Solid Edge part; units mm, degrees
sketch "Sketch1" plane through (0, 0, 0) normal (0, 0, 1) x (1, 0, 0)
  circle A0 centre (0, 0) radius 6
extrude "Protrusion1" add sketch "Sketch1" along normal mid plane 30
sketch "Sketch2" plane through (0, 0, 15) normal (0, 0, 1) x (1, 0, 0)
  line L0 (-9.9593, 5.75) -> (-9.9593, -5.75)
  line L1 (-9.9593, -5.75) -> (0, -11.5)
  line L2 (0, -11.5) -> (9.9593, -5.75)
  line L3 (9.9593, -5.75) -> (9.9593, 5.75)
  line L4 (9.9593, 5.75) -> (0, 11.5)
  line L5 (0, 11.5) -> (-9.9593, 5.75)
extrude "Protrusion2" add sketch "Sketch2" along normal blind 10
chamfer "Chamfer1" distance 1 angle 45 1 edges at (-6, 0, -15)
properties material "알루미늄, 1060"
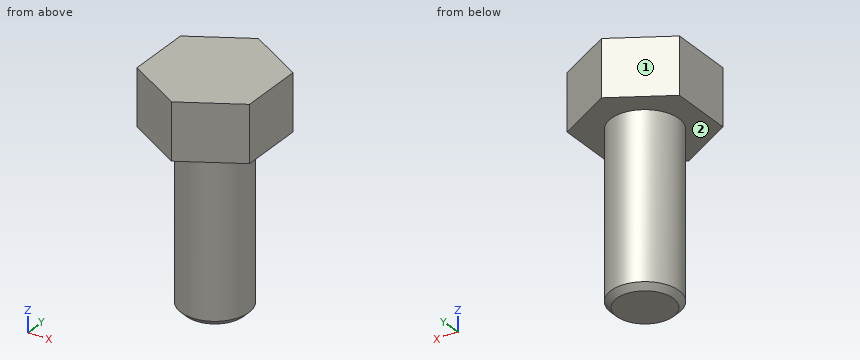
Geometry check sheet. Reference: the model listing, model coordinates, mm. Face numbers are marked on the shaded views. A direction names the side the tool comes from. Give positions to 0.01 mm unless a question says otherwise; leave off trailing zeros. Write each loop counter-clockwise with the first axis right and the second up, starting at its lowest first coordinate (ties: lowest second). Pieces come first, ordered by that corner, then holes.
1) Cross-section at C-C (x = 8.5). Record the boundary of the cut face in (y, z).
Values follow:
outline: (-6.59, 15) - (6.59, 15) - (6.59, 25) - (-6.59, 25) - close
2) Set-up check for the marked faces 1 and 2: record each of +Z, -Z, +X, -X, +Y, -Y from which the full face is reachable in a straight line by a thin tool's end or side.
Values follow:
face 1: +Z, -Z, -X, +Y
face 2: -Z
3) Cross-section at A-A (y = 0). Record the boundary of the cut face in (x, z).
Values follow:
outline: (-9.96, 15) - (-6, 15) - (-6, -14) - (-5, -15) - (5, -15) - (6, -14) - (6, 15) - (9.96, 15) - (9.96, 25) - (-9.96, 25) - close
4) Thickness scan on line 1 (Z direction, x = -8, y = 4.25); line 2 (Y direction, x = 4.5, z = -6); line 3 (X direction, y = 2.5, z = 1.5). Record the ranges inside material, lowest first.
Values follow:
line 1: z = 15 to 25
line 2: y = -3.97 to 3.97
line 3: x = -5.45 to 5.45
5) Go/stop test with flat-tipped pins: pin 1 Ø1 at (y, z) = (1.5, 2) entering from +X; pin 2 Ø3 at (x, z) = (1, -5.5) entering from -Y; pin 3 Ø6 at (y, z) = (6, -0.5) entering from +X. Record where each tip stops, or that it passes through.
Values follow:
pin 1: stops at x = 5.92
pin 2: stops at y = -6
pin 3: stops at x = 5.2
6) Cross-section at B-B (z = 6.5). Record the boundary of the cut face in (x, y).
Values follow:
outline: circle Ø12 at (0, 0)
7) Cross-section at D-D (y = 7). Record the boundary of the cut face in (x, z).
Values follow:
outline: (-7.79, 15) - (7.79, 15) - (7.79, 25) - (-7.79, 25) - close
